CAD build for the part. Positions are in the model's coordinates, mm. A direction names the side the tool comes from. Give positions to 0.01 mm unless a question says otherwise; leave off trailing zeros. Write each loop counter-clockwise with the first axis right and the second up, starting at its lowest first coordinate (ties: lowest second). Pieces come first, ordered by that corner, then holes. Notation, with made-up numbers: (74, 44.25) - (81, 44.25) arc R32 ccw to (81, 77.25) - close; hole circle Ø1 at (10.25, -36). An arc over 180 degrees is marked (long way). Write item = value, one per line. Start each with the question number.
```python
from build123d import *

# Parameters (mm, degrees)
BOSS_EXTRUDE1_DEPTH = 82.55
CUT_EXTRUDE1_REACH  = 139.687
CUT_EXTRUDE2_REACH  = 139.687
SKETCH3_R           = 3.97
SKETCH5_R           = 4.15
CUT_EXTRUDE4_DEPTH  = 1
CUT_EXTRUDE5_REACH  = 191.559
SKETCH6_R           = 1.6
CHAMFER1_SIZE       = 2
CHAMFER2_SIZE       = 1
SKETCH7_W           = 165.1
SKETCH7_H           = 2
CUT_EXTRUDE6_DEPTH  = 1.5


with BuildPart() as part:
    # Sketch1 → Boss-Extrude1 (new, symmetric)
    with BuildSketch(Plane(origin=(0, 0, 0), x_dir=(0, 0, -1), z_dir=(1, 0, 0))):
        with BuildLine():
            Line((-80, -33.521656958), (-80, 10.521656958))
            ThreePointArc((-80, 10.521656958), (-70.712477852, 30.438812479), (-49.485147381, 36.126658537))
            Line((-49.485147381, 36.126658537), (58.514852619, 17.08334462))
            ThreePointArc((58.514852619, 17.08334462), (73.917155521, 8.190820894), (80, -8.521656958))
            Line((80, -8.521656958), (80, -33.521656958))
            Line((80, -33.521656958), (68, -33.521656958))
            Line((68, -33.521656958), (68, -36.521656958))
            Line((68, -36.521656958), (80, -36.521656958))
            ThreePointArc((80, -36.521656958), (82.121320344, -35.642977302), (83, -33.521656958))
            Line((83, -33.521656958), (83, -8.521656958))
            ThreePointArc((83, -8.521656958), (76.21528885, 10.119183723), (59.035797152, 20.037767879))
            Line((59.035797152, 20.037767879), (-48.964202848, 39.081081796))
            ThreePointArc((-48.964202848, 39.081081796), (-72.640840681, 32.736945809), (-83, 10.521656958))
            Line((-83, 10.521656958), (-83, -33.521656958))
            ThreePointArc((-83, -33.521656958), (-82.121320344, -35.642977302), (-80, -36.521656958))
            Line((-80, -36.521656958), (-68, -36.521656958))
            Line((-68, -36.521656958), (-68, -33.521656958))
            Line((-68, -33.521656958), (-80, -33.521656958))
        make_face()
    extrude(amount=BOSS_EXTRUDE1_DEPTH, both=True)

    # Sketch2 → Cut-Extrude1 (cut, up to next)
    with BuildSketch(Plane(origin=(0, 29.529271148, -5.206807224), x_dir=(1, 0, 0), z_dir=(0, 0.984807753012209, -0.1736481776669248)), mode=Mode.PRIVATE) as cut_extrude1_sk1:
        with BuildLine():
            Line((-16, -8.440611136), (46, -8.440611136))
            ThreePointArc((46, -8.440611136), (47.060660172, -8.001271308), (47.5, -6.940611136))
            Line((47.5, -6.940611136), (47.5, 28.159388864))
            ThreePointArc((47.5, 28.159388864), (47.060660172, 29.220049036), (46, 29.659388864))
            Line((46, 29.659388864), (-16, 29.659388864))
            ThreePointArc((-16, 29.659388864), (-17.060660172, 29.220049036), (-17.5, 28.159388864))
            Line((-17.5, 28.159388864), (-17.5, -6.940611136))
            ThreePointArc((-17.5, -6.940611136), (-17.060660172, -8.001271308), (-16, -8.440611136))
        make_face()
    cut_extrude1_tool1 = extrude(cut_extrude1_sk1.sketch, amount=-CUT_EXTRUDE1_REACH, mode=Mode.PRIVATE) & part.part
    add(cut_extrude1_tool1.solids().sort_by_distance((15, 27.68697, -15.655016))[0], mode=Mode.SUBTRACT)

    # Sketch3 → Cut-Extrude2 (cut, up to next)
    with BuildSketch(Plane(origin=(0, 29.529271148, -5.206807224), x_dir=(1, 0, 0), z_dir=(0, 0.984807753012209, -0.1736481776669248)), mode=Mode.PRIVATE) as cut_extrude2_sk1:
        with Locations(Location((49.2, -31.254272732, 0), (0, 0, 270))):
            Circle(SKETCH3_R)
    cut_extrude2_tool1 = extrude(cut_extrude2_sk1.sketch, amount=-CUT_EXTRUDE2_REACH, mode=Mode.PRIVATE) & part.part
    # Sketch3 → Cut-Extrude2 (cut, up to next)
    with BuildSketch(Plane(origin=(0, 29.529271148, -5.206807224), x_dir=(1, 0, 0), z_dir=(0, 0.984807753012209, -0.1736481776669248)), mode=Mode.PRIVATE) as cut_extrude2_sk2:
        with Locations(Location((30.15, -31.254272732, 0), (0, 0, 270))):
            Circle(SKETCH3_R)
    cut_extrude2_tool2 = extrude(cut_extrude2_sk2.sketch, amount=-CUT_EXTRUDE2_REACH, mode=Mode.PRIVATE) & part.part
    # Sketch3 → Cut-Extrude2 (cut, up to next)
    with BuildSketch(Plane(origin=(0, 29.529271148, -5.206807224), x_dir=(1, 0, 0), z_dir=(0, 0.984807753012209, -0.1736481776669248)), mode=Mode.PRIVATE) as cut_extrude2_sk3:
        with BuildLine():
            Line((-64.777738917, -18.950611136), (-65.05, -18.950611136))
            ThreePointArc((-65.05, -18.950611136), (-65.757106781, -19.243504355), (-66.05, -19.950611136))
            Line((-66.05, -19.950611136), (-66.05, -20.350611136))
            ThreePointArc((-66.05, -20.350611136), (-65.757106781, -21.057717917), (-65.05, -21.350611136))
            Line((-65.05, -21.350611136), (-64.777738917, -21.350611136))
            ThreePointArc((-64.777738917, -21.350611136), (-44.85, -20.150611136), (-64.777738917, -18.950611136))
        make_face()
    cut_extrude2_tool3 = extrude(cut_extrude2_sk3.sketch, amount=-CUT_EXTRUDE2_REACH, mode=Mode.PRIVATE) & part.part
    add(cut_extrude2_tool1.solids().sort_by_distance((49.2, 34.956519, 25.572643))[0], mode=Mode.SUBTRACT)
    add(cut_extrude2_tool2.solids().sort_by_distance((30.15, 34.956519, 25.572643))[0], mode=Mode.SUBTRACT)
    add(cut_extrude2_tool3.solids().sort_by_distance((-54.933345, 33.028388, 14.637671))[0], mode=Mode.SUBTRACT)

    # Sketch5 → Cut-Extrude4 (cut)
    with BuildSketch(Plane(origin=(0, 26.574847889, -4.685862691), x_dir=(1, 0, 0), z_dir=(0, -0.984807753012209, 0.1736481776669249))):
        with Locations(Location((57.15, -23.759388864, 0), (0, 0, 270))):
            Circle(SKETCH5_R)
        with Locations(Location((-28.95, -23.759388864, 0), (0, 0, 270))):
            Circle(SKETCH5_R)
        with Locations(Location((-28.95, 7.990611136, 0), (0, 0, 270))):
            Circle(SKETCH5_R)
        with Locations(Location((57.15, 7.990611136, 0), (0, 0, 270))):
            Circle(SKETCH5_R)
    extrude(amount=-CUT_EXTRUDE4_DEPTH, mode=Mode.SUBTRACT)

    # Sketch6 → Cut-Extrude5 (cut, up to next)
    with BuildSketch(Plane.XY.offset(83), mode=Mode.PRIVATE) as cut_extrude5_sk1:
        with Locations((79.225, -16.196656958)):
            Circle(SKETCH6_R)
    cut_extrude5_tool1 = extrude(cut_extrude5_sk1.sketch, amount=-CUT_EXTRUDE5_REACH, mode=Mode.PRIVATE) & part.part
    # Sketch6 → Cut-Extrude5 (cut, up to next)
    with BuildSketch(Plane.XY.offset(83), mode=Mode.PRIVATE) as cut_extrude5_sk2:
        with Locations((55.225, -7.196656958)):
            Circle(SKETCH6_R)
    cut_extrude5_tool2 = extrude(cut_extrude5_sk2.sketch, amount=-CUT_EXTRUDE5_REACH, mode=Mode.PRIVATE) & part.part
    # Sketch6 → Cut-Extrude5 (cut, up to next)
    with BuildSketch(Plane.XY.offset(83), mode=Mode.PRIVATE) as cut_extrude5_sk3:
        with BuildLine():
            Line((60.45, -4.421656958), (74.05, -4.421656958))
            ThreePointArc((74.05, -4.421656958), (75.110660172, -4.860996786), (75.55, -5.921656958))
            Line((75.55, -5.921656958), (75.55, -17.521656958))
            ThreePointArc((75.55, -17.521656958), (75.110660172, -18.58231713), (74.05, -19.021656958))
            Line((74.05, -19.021656958), (60.45, -19.021656958))
            ThreePointArc((60.45, -19.021656958), (59.389339828, -18.58231713), (58.95, -17.521656958))
            Line((58.95, -17.521656958), (58.95, -5.921656958))
            ThreePointArc((58.95, -5.921656958), (59.389339828, -4.860996786), (60.45, -4.421656958))
        make_face()
    cut_extrude5_tool3 = extrude(cut_extrude5_sk3.sketch, amount=-CUT_EXTRUDE5_REACH, mode=Mode.PRIVATE) & part.part
    add(cut_extrude5_tool1.solids().sort_by_distance((79.225, -16.196657, 83))[0], mode=Mode.SUBTRACT)
    add(cut_extrude5_tool2.solids().sort_by_distance((55.225, -7.196657, 83))[0], mode=Mode.SUBTRACT)
    add(cut_extrude5_tool3.solids().sort_by_distance((67.25, -11.721657, 83))[0], mode=Mode.SUBTRACT)

    # Chamfer1
    chamfer1_edges = [part.edges().sort_by_distance(p)[0] for p in [
        (47.060660172, 24.455262881, -33.982938058),
        (15, 24.378972321, -34.415603327),
        (-17.060660172, 24.455262881, -33.982938058),
        (-17.5, 27.686970105, -15.655015632),
        (-17.060660172, 30.918677329, 2.672906794),
        (15, 30.99496789, 3.105572063),
        (47.060660172, 30.918677329, 2.672906794),
        (47.5, 27.686970105, -15.655015632),
    ]]
    chamfer(chamfer1_edges, length=CHAMFER1_SIZE)

    # Chamfer2
    chamfer2_edges = [part.edges().sort_by_distance(p)[0] for p in [
        (49.2, 34.267135387, 21.662956098),
        (30.15, 34.267135387, 21.662956098),
    ]]
    chamfer(chamfer2_edges, length=CHAMFER2_SIZE)

    # Sketch7 → Cut-Extrude6 (cut)
    with BuildSketch(Plane.XZ.offset(36.521656958)):
        with Locations((0, 69)):
            Rectangle(SKETCH7_W, SKETCH7_H)
        with Locations((0, -69)):
            Rectangle(SKETCH7_W, SKETCH7_H)
    extrude(amount=-CUT_EXTRUDE6_DEPTH, mode=Mode.SUBTRACT)


solid = part.part
```
1. Mould opens along X. For faces 5 (the flat face through (-18.49, 26.65, -15.72)), 6 (the cylindrical face through (1.156, 8.385, -73.753)) say: +X half, -X half, draft (parallel to the pull), parting line (faces both ways), or undercut.
2. Cut at B-B (y = 6). Give the cut face in (x, z).
3. Cut at C-C (z = -61.5). Give the cut face in (x, y).
4. Tool access for faces 1 (the flat face through (47.5, 25, -15)), 2 (the flat face through (1, -11, 83)), 3 (the flat face through (1.156, 28.854, 8.241)), 4 (the flat face through (1, -12, 80)): list every direction of +Z, -Z, +X, -X, +Y, -Y with a clear straight run to the whole face (end or side of a thin tool).
5. Wall check: line 1 along Z through (x, y) = (20, -17); line 2 along Y through (x, z) = (-45.5, 73); line 3 along Z through (x, y) = (-35.5, 1.5). Give the ranges that are in metal, low to high.
6. Cut at A-A (x = 2). Give the cut face in (y, z).
7. Pin check, flat tips, straight feed: pin 1 Ø1.6 at (x, y) = (6, -34.5) entering from +Z; pin 2 Ø3.5 at (x, z) = (69.5, 82) entering from -Y; pin 3 Ø1.2 at (x, y) = (15.5, -36) entering from -Z. Stop position of each tip, or through.
Output:
q1.face_5 = undercut
q1.face_6 = draft
q2.outline = (-82.55, -79.1) - (82.55, -79.1) - (82.55, -75.57) - (-82.55, -75.57) - close; (-82.55, 80) - (82.55, 80) - (82.55, 83) - (-82.55, 83) - close
q3.outline = (-82.55, 16.37) - (82.55, 16.37) - (82.55, 19.49) - (-82.55, 19.49) - close
q4.face_1 = +Y, -Y
q4.face_2 = +Z, +X, -X, +Y, -Y
q4.face_3 = +X, -X, -Y
q4.face_4 = +X, -X
q5.line_1 = -83 to -80, 80 to 83
q5.line_2 = -36.52 to -33.52, 28.27 to 32.43
q5.line_3 = -81.21 to -77.99, 80 to 83
q6.outline = (-36.52, -80) arc R3 ccw to (-33.52, -83) - (-8.52, -83) arc R29 ccw to (20.04, -59.04) - (24.03, -36.39) - (22.41, -34.07) - (21.42, -33.89) - (17.08, -58.51) arc R26 cw to (-8.52, -80) - (-33.52, -80) - (-33.52, -68) - (-35.02, -68) - (-35.02, -70) - (-36.52, -70) - close; (-36.52, 70) - (-35.02, 70) - (-35.02, 68) - (-33.52, 68) - (-33.52, 80) - (10.52, 80) arc R26 cw to (36.13, 49.49) - (28.04, 3.63) - (29.03, 3.45) - (31.34, 5.08) - (39.08, 48.96) arc R29 ccw to (10.52, 83) - (-33.52, 83) arc R3 ccw to (-36.52, 80) - close
q7.pin_1 = 82.99
q7.pin_2 = -36.51
q7.pin_3 = -82.34
